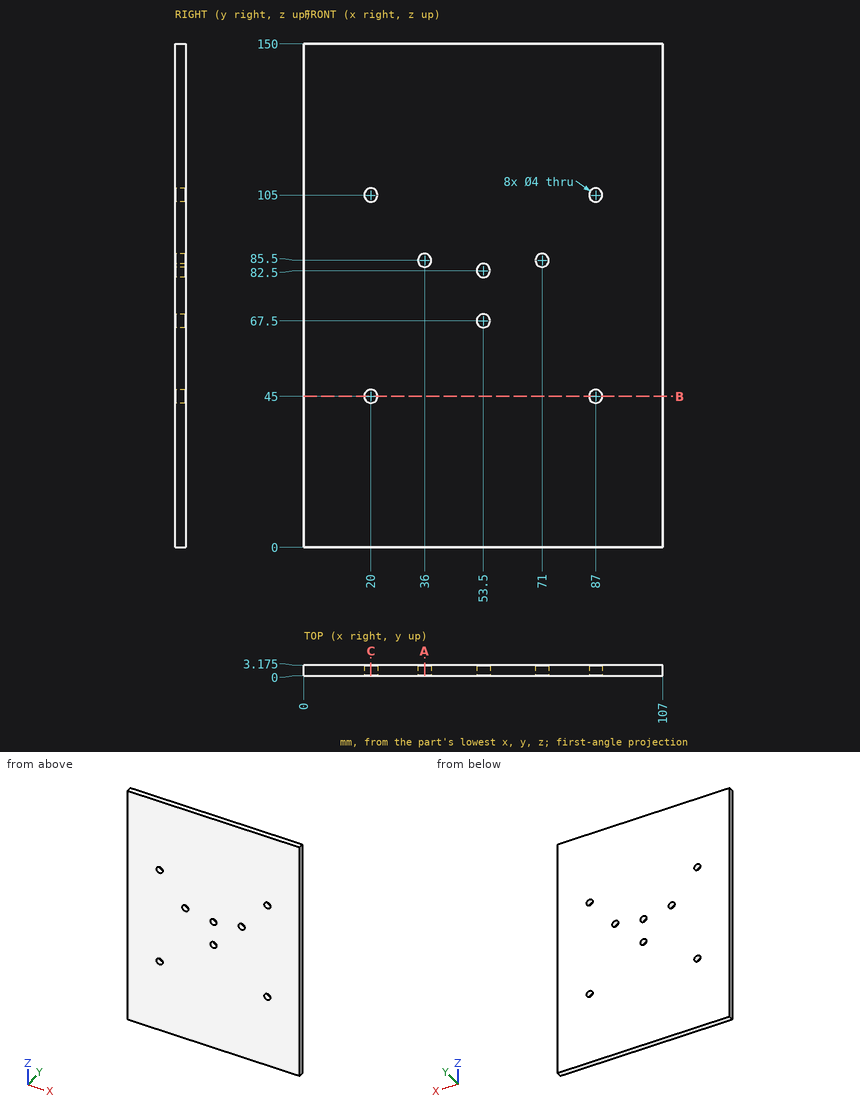
Here's the drawing with two shaded views (mm, measured from the low corner). I have some questions. Round coordinates to 2 decimals unless told otherwise and drop trailing zeros. Loops run counter-clockwise (first coordinate to the right, second up) from the corner with the lowest first, then second, coordinate; pieces in that order, holes last.
1. Suppose I cut it at C-C, the plane x = 20. Please give me the cut outline in (y, z) (3 decimals), and give its area (3 significant figures).
Answers:
outline: (0, 0) - (3.175, 0) - (3.175, 43) - (0, 43) - close; (0, 47) - (3.175, 47) - (3.175, 103) - (0, 103) - close; (0, 107) - (3.175, 107) - (3.175, 150) - (0, 150) - close
area: 451 mm2
2. Suppose I cut it at A-A, the plane x = 36. Please give me the cut outline in (y, z) (3 decimals).
Answers:
outline: (0, 0) - (3.175, 0) - (3.175, 83.5) - (0, 83.5) - close; (0, 87.5) - (3.175, 87.5) - (3.175, 150) - (0, 150) - close
3. Suppose I cut it at B-B, the plane z = 45. Please give me the cut outline in (x, y) (3 decimals).
Answers:
outline: (0, 0) - (18, 0) - (18, 3.175) - (0, 3.175) - close; (22, 0) - (85, 0) - (85, 3.175) - (22, 3.175) - close; (89, 0) - (107, 0) - (107, 3.175) - (89, 3.175) - close
4. If I drill on probe 1 along Z at (x, y) = (87, 1.65); probe 2 along X at (y, z) = (1.7, 105); probe 3 along Z at (x, y) = (54, 2.8), over which ranges is the centre line in solid material (lowest first)?
Answers:
probe 1: z = 0 to 43, 47 to 103, 107 to 150
probe 2: x = 0 to 18, 22 to 85, 89 to 107
probe 3: z = 0 to 65.56, 69.44 to 80.56, 84.44 to 150
